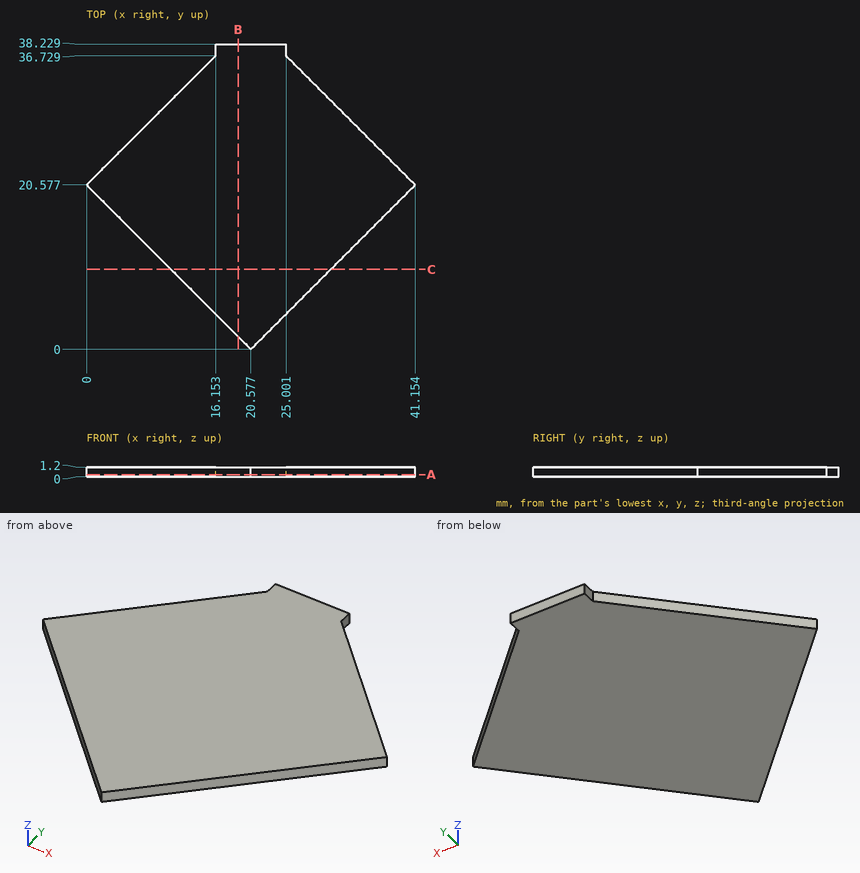
Could you check a few things on this drawing? It's one solid part, dimensions in mm from its lowest x, y, z. Coordinates: 2 decimals unless noted, no trailing zeros. Loops run counter-clockwise (first coordinate to the right, second up) from the corner with the lowest first, then second, coordinate; pieces in that order, holes last.
1. Imagine slicing it at A-A (z = 0.3). Please give me the cut outline in (x, y).
2. Imagine slicing it at C-C (y = 10). Please give me the cut outline in (x, z).
3. For P1, Ø2, axis at x = 23, y = 18, coming from the -Z side, with a flat end and sliding along its axis, tell me the tip position at first contact or that it passes through.
4. I need wall thicknesses on L1, parallel to X at y = 19.5, z = 0.7 (1 decimal); L2, parallel to Y at x = 36, z = 0.25 (1 decimal). Which ranges of each line are inside material? Lowest first, please.
5. Imagine slicing it at B-B (x = 19). Please give me the cut outline in (y, z).
Computed values:
1. outline: (0, 20.58) - (20.58, 0) - (41.15, 20.58) - (25, 36.73) - (25, 38.23) - (16.15, 38.23) - (16.15, 36.73) - close
2. outline: (10.58, 0) - (30.58, 0) - (30.58, 1.2) - (10.58, 1.2) - close
3. P1: stops at z = 0
4. L1: x = 1.1 to 40.1
4. L2: y = 15.4 to 25.7
5. outline: (1.58, 0) - (38.23, 0) - (38.23, 1.2) - (1.58, 1.2) - close
